The figure shows three views and two pictorial views of one solid part (mm, origin at its lowest corner). Answer the questions. Coordinates: 2 decimals unless noted, no trailing zeros. Loops run counter-clockwise (first coordinate to the right, second up) from the corner with the lowest first, then second, coordinate; pieces in that order, holes last. Notation, with made-up numbers: M 49.5,-7 L 95.5,-7 A6 ccw 95.5,2 Z; hole C -20.5,-7.75 d7. An arc over 180 degrees is marked long. Return JSON: item names as keys, results as strings. Group by question number.
1. Given P1, Ø3, axis at y = 31.5, z = 11, coming from the -X side; P2, Ø1.5, axis at y = 59, z = 6, coming from the +X side; P3, Ø1, axis at x = 44, z = 11, coming from the +Y side, each flat-ended and moving along its own axis, determine where each tip first touches the part or whether it passes through.
2. Section B-B (x = 146.05) is taken. Write down the section's boundary in (y, z) (1 decimal).
3. Straight lines are drawn through the part: L1, parallel to Y at x = 6.35, z = 1.9; L2, parallel to Y at x = 133, z = 2.25; L3, parallel to Y at x = 146.05, z = 1.7. For each, find the intervals that lie inside material, in ascending order. Write a range as from..to.
4. The mould has two halves that part along Y. Classify the marked faces 1, 2 and 3: pulls with the +Y half, pulls with the -Y half, needs draft (parallel to the pull), parting line crosses it, or undercut.
5. Section D-D (y = 44.5) is taken. Write down the section's boundary in (x, z) (1 decimal).
6. Section A-A (x = 6.35) is taken. Write down the section's boundary in (y, z) (1 decimal).
7. Section C-C (z = 7) is taken. Write down the section's boundary in (x, y).
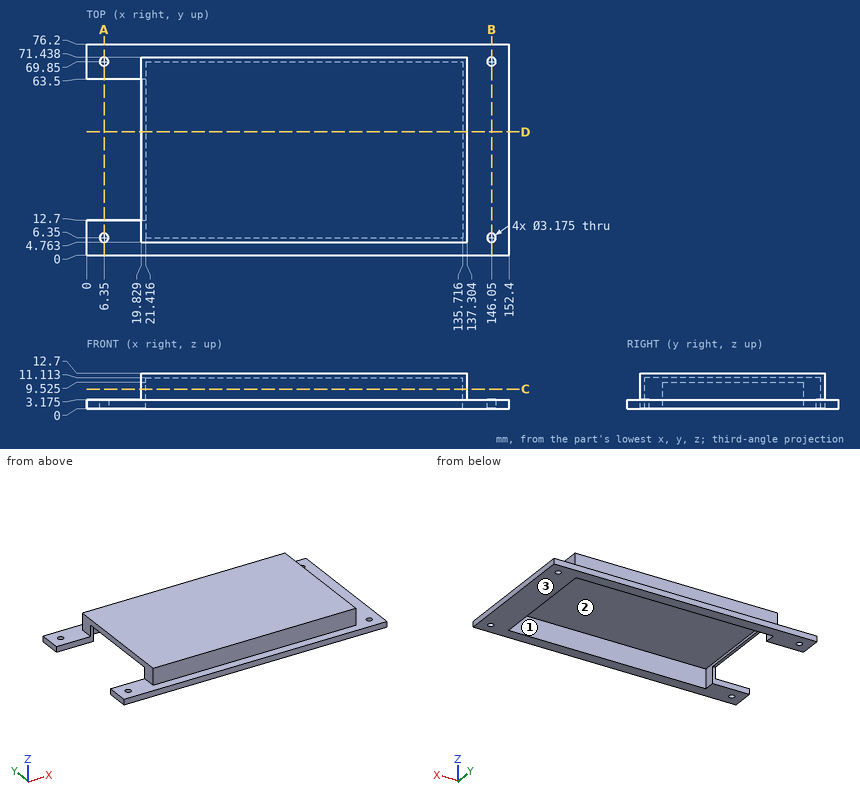
Worked out:
{
 "1": {"P1": "x = 19.83", "P2": "x = 137.3", "P3": "y = 71.44"},
 "2": {"outline": "M 0,0 L 4.8,0 L 4.8,3.2 L 0,3.2 Z; M 7.9,0 L 68.3,0 L 68.3,3.2 L 7.9,3.2 Z; M 71.4,0 L 76.2,0 L 76.2,3.2 L 71.4,3.2 Z"},
 "3": {"L1": "0..4.76, 7.94..12.7, 63.5..68.26, 71.44..76.2", "L2": "0..6.35, 69.85..76.2", "L3": "0..4.76, 7.94..68.26, 71.44..76.2"},
 "4": {"face 1": "undercut", "face 2": "undercut", "face 3": "needs draft"},
 "5": {"outline": "M 19.8,9.5 L 21.4,9.5 L 21.4,11.1 L 135.7,11.1 L 135.7,0 L 152.4,0 L 152.4,3.2 L 137.3,3.2 L 137.3,12.7 L 19.8,12.7 Z"},
 "6": {"outline": "M 0,0 L 4.8,0 L 4.8,3.2 L 0,3.2 Z; M 7.9,0 L 12.7,0 L 12.7,3.2 L 7.9,3.2 Z; M 63.5,0 L 68.3,0 L 68.3,3.2 L 63.5,3.2 Z; M 71.4,0 L 76.2,0 L 76.2,3.2 L 71.4,3.2 Z"},
 "7": {"outline": "M 19.83,4.76 L 137.3,4.76 L 137.3,71.44 L 19.83,71.44 L 19.83,63.5 L 21.42,63.5 L 21.42,69.85 L 135.72,69.85 L 135.72,6.35 L 21.42,6.35 L 21.42,12.7 L 19.83,12.7 Z"}
}
